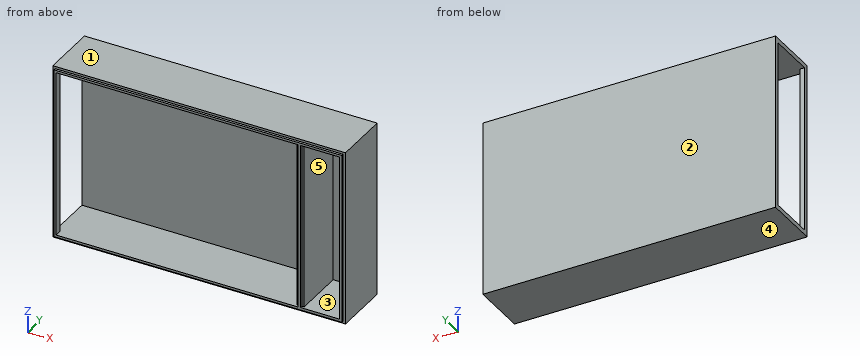
```python
from build123d import *

# Parameters (mm, degrees)
F0_W      = 127
F0_H      = 76.2
F1_DEPTH  = 25.4
F2_W      = 15.9999934
F2_H      = 72.136
F3_DEPTH  = 23.4188
F4_W      = 0.9906
F4_H      = 72.136
F5_DEPTH  = 0.9906
F6_W      = 127
F6_H      = 0.9906
F7_DEPTH  = 0.9906
F8_W      = 0.9906
F8_H      = 75.2094
F9_DEPTH  = 0.9906
F10_W     = 0.9906
F10_H     = 75.2094
F11_DEPTH = 0.9906
F12_W     = 125.0188
F12_H     = 0.9906
F13_DEPTH = 0.9906
F14_W     = 104.0658066
F14_H     = 72.2376
F15_DEPTH = 23.4188
F16_W     = 0.9906
F16_H     = 72.2376
F17_DEPTH = 0.9906
F18_W     = 20.447
F18_H     = 72.2376
F19_DEPTH = 1.9812


with BuildPart() as f1:
    # F0 (on Front) → F1 (new body)
    with BuildSketch(Plane.XZ):
        Rectangle(F0_W, F0_H)
    extrude(amount=F1_DEPTH)

    # F2 (on face) → F3 (cut)
    with BuildSketch(Plane.XZ.offset(25.4)):
        with Locations((53.5188033, 0.0508)):
            Rectangle(F2_W, F2_H)
    extrude(amount=-F3_DEPTH, mode=Mode.SUBTRACT)

    # F4 (on face) → F5 (cut)
    with BuildSketch(Plane.XZ.offset(25.4)):
        with Locations((45.0235066, 0.0508)):
            Rectangle(F4_W, F4_H)
    extrude(amount=-F5_DEPTH, mode=Mode.SUBTRACT)

    # F6 (on face) → F7 (cut)
    with BuildSketch(Plane.XZ.offset(25.4)):
        with Locations((0, 37.6047)):
            Rectangle(F6_W, F6_H)
    extrude(amount=-F7_DEPTH, mode=Mode.SUBTRACT)

    # F8 (on face) → F9 (cut)
    with BuildSketch(Plane.XZ.offset(25.4)):
        with Locations((63.0047, -0.4953)):
            Rectangle(F8_W, F8_H)
    extrude(amount=-F9_DEPTH, mode=Mode.SUBTRACT)

    # F10 (on face) → F11 (cut)
    with BuildSketch(Plane.XZ.offset(25.4)):
        with Locations((-63.0047, -0.4953)):
            Rectangle(F10_W, F10_H)
    extrude(amount=-F11_DEPTH, mode=Mode.SUBTRACT)

    # F12 (on face) → F13 (cut)
    with BuildSketch(Plane.XZ.offset(25.4)):
        with Locations((0, -37.6047)):
            Rectangle(F12_W, F12_H)
    extrude(amount=-F13_DEPTH, mode=Mode.SUBTRACT)

    # F14 (on face) → F15 (cut)
    with BuildSketch(Plane.XZ.offset(25.4)):
        with Locations((-9.4858967, 0)):
            Rectangle(F14_W, F14_H)
    extrude(amount=-F15_DEPTH, mode=Mode.SUBTRACT)

    # F16 (on face) → F17 (cut)
    with BuildSketch(Plane.XZ.offset(25.4)):
        with Locations((43.0423066, 0)):
            Rectangle(F16_W, F16_H)
    extrude(amount=-F17_DEPTH, mode=Mode.SUBTRACT)

    # F18 (on face) → F19 (cut)
    with BuildSketch(Plane(origin=(-63.5, 0, 0), x_dir=(0, -1, 0), z_dir=(-1, 0, 0))):
        with Locations((12.2047, 0)):
            Rectangle(F18_W, F18_H)
    extrude(amount=-F19_DEPTH, mode=Mode.SUBTRACT)


solid = f1.part
```
Source: CAD feature listing. Evaluate the final solid. Frame: model axes, mm. Face numbers are marked on the shaded views. A direction names the side the tool comes from. Round coordinates to 2 decimals unless told otherwise and drop trailing zeros. Order: outer loops, then holes, each group sorted by start corner. A loop starts at its lowest first (then second) coordinate and runs counter-clockwise, first axis right, second up. Notation, with made-up numbers: (68, 33) -> (84, 33) arc R17 ccw to (84, 49) -> close; hole circle Ø3 at (48, 2). An arc over 180 degrees is marked (long way). One line per item, written item: value. Start each with the question number.
Q1. Section query B-B (y = -3.5). Return the cut outline in (x, z), plus the area to 3 significant figures.
Q2. Material intervals for probe 1 along X at (y, z) = (-20, 14); probe 2 along Z at (x, y) = (27, -14); probe 3 along Y at (x, z) = (34.5, -15), sorted ascending.
Q3. Access query for the marked faces 4 and 5. Directions: +Z, -Z, +X, -X, +Y, -Y. A direction counts if a zero-diameter tool reaches every point of the face in a straight line with its end or side. Return the directions, or none.
Q4. Draft query along Z for the marked faces 1, 2 and 3. Return one class per face: pulls with the +Z half, pulls with the -Z half, needs draft (parallel to the pull), parting line crosses it, or undercut.
Q5. Section query A-A (z = 25). Return the cut outline in (x, y), plus the area to 3 significant figures.
Q6. Section query C-C (x = 26). Return the cut outline in (y, z).
Q7. Pin query (flat end, axial travel): pin 1 (1 mm diameter, centred on y = -3.5, z = 5.5, fed in from -X); pin 2 (1.1 mm diameter, centred on y = -25, z = -17, fed in from -X); pin 3 (8 mm diameter, centred on x = 9.5, z = -26.5, fed in from -Y). Return the tip coordinate at first contact, or that it passes through.
Findings below:
1. outline: (-63.5, -38.1) -> (63.5, -38.1) -> (63.5, 38.1) -> (-63.5, 38.1) -> (-63.5, 36.12) -> (42.55, 36.12) -> (42.55, -36.12) -> (-63.5, -36.12) -> close; hole (45.52, -36.02) -> (61.52, -36.02) -> (61.52, 36.12) -> (45.52, 36.12) -> close
1. area: 863 mm²
2. probe 1: 42.55 to 45.52, 61.52 to 63.5
2. probe 2: -38.1 to -36.12, 36.12 to 38.1
2. probe 3: -1.98 to 0
3. face 4: -Z, +X, -X, +Y, -Y
3. face 5: -Y
4. face 1: pulls with the +Z half
4. face 2: needs draft
4. face 3: undercut
5. outline: (-63.5, -24.41) -> (-62.51, -24.41) -> (-62.51, -25.4) -> (-61.52, -25.4) -> (-61.52, -22.43) -> (-63.5, -22.43) -> close; (-63.5, -1.98) -> (42.55, -1.98) -> (42.55, -24.41) -> (43.54, -24.41) -> (43.54, -25.4) -> (44.53, -25.4) -> (44.53, -24.41) -> (45.52, -24.41) -> (45.52, -1.98) -> (61.52, -1.98) -> (61.52, -25.4) -> (62.51, -25.4) -> (62.51, -24.41) -> (63.5, -24.41) -> (63.5, 0) -> (-63.5, 0) -> close
5. area: 370 mm²
6. outline: (-25.4, -37.11) -> (-24.41, -37.11) -> (-24.41, -38.1) -> (0, -38.1) -> (0, 38.1) -> (-24.41, 38.1) -> (-24.41, 37.11) -> (-25.4, 37.11) -> (-25.4, 36.12) -> (-1.98, 36.12) -> (-1.98, -36.12) -> (-25.4, -36.12) -> close
7. pin 1: x = 42.55
7. pin 2: x = -62.51
7. pin 3: y = -1.98
